```python
from build123d import *

# Parameters (mm, degrees)
SKETCH4_R               = 0.5
CUT_EXTRUDE1_DEPTH      = 60
CUT_EXTRUDE2_DEPTH      = 65.078926224
CUT_EXTRUDE2_DEPTH_BACK = 65.078926224
SKETCH5_R               = 2.5


with BuildPart() as part:
    # Sketch3 → Revolve1 (revolve)
    with BuildSketch(Plane.XY):
        with BuildLine():
            Line((-1.903971709, 4.611227449), (60.096028291, 4.611227449))
            Line((60.096028291, 4.611227449), (63.096028291, 1.611227449))
            Line((63.096028291, 1.611227449), (63.096028291, -0.388772551))
            Line((63.096028291, -0.388772551), (-6.903971709, -0.388772551))
            ThreePointArc((-6.903971709, -0.388772551), (-5.439505615, 3.146761355), (-1.903971709, 4.611227449))
        make_face()
    revolve(axis=Axis((63.096028291, -0.388772551, 0), (-1, 0, 0)))

    # Sketch4 → Cut-Extrude1 (cut)
    with BuildSketch(Plane(origin=(63.096028291, 0, 0), x_dir=(0, 0, -1), z_dir=(1, 0, 0))):
        with Locations(Location((0, -0.388772551, 0), (0, 0, 90))):
            Circle(SKETCH4_R)
    extrude(amount=-CUT_EXTRUDE1_DEPTH, mode=Mode.SUBTRACT)

    # Sketch5 → Cut-Extrude2 (cut, two sides: drawn at the far end of the back side and taken through both)
    with BuildSketch(Plane(origin=(0, 4.611227449, 0), x_dir=(1, 0, 0), z_dir=(0, 1, 0)).offset(-CUT_EXTRUDE2_DEPTH_BACK)):
        with Locations(Location((55.096028291, 0, 0), (0, 0, 180))):
            Circle(SKETCH5_R)
    extrude(amount=CUT_EXTRUDE2_DEPTH + CUT_EXTRUDE2_DEPTH_BACK, mode=Mode.SUBTRACT)


solid = part.part
```
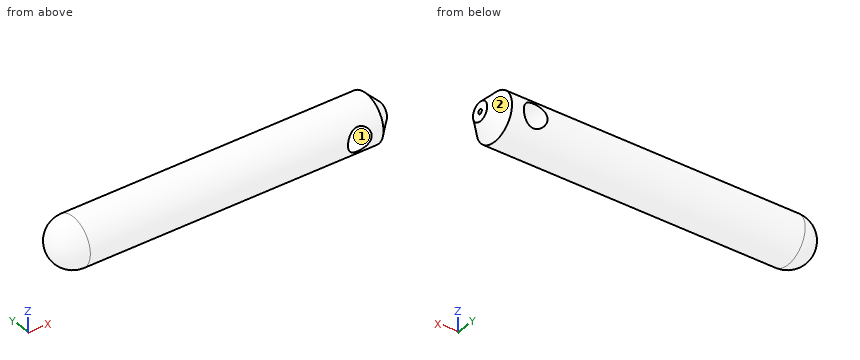
For this review, take the finished solid that the model builds, in its own axes (mm). Face numbers are marked on the shaded views. Round coordinates to 2 decimals unless told otherwise and drop trailing zeros. Write each loop counter-clockwise with the first axis right and the second up, starting at its lowest first coordinate (ties: lowest second). Pieces come first, ordered by that corner, then holes. Notation, with made-up numbers: (-3, 45) - (46, 45) arc R3 cw to (46, 50) - close; hole circle Ø1 at (18.25, 52). An arc over 180 degrees is marked (long way). Answer as a JSON object with one key per item and string values.
1. To check wall thickness, follow line 1 along Y through (x, z) = (7, 0); line 2 along X through (y, z) = (3.25, -0.25); line 3 along X through (y, z) = (2, 0.5). State the ranges of each line that lie inside material, in increasing order.
Response values:
{"line 1": "y = -5.39 to -0.89, 0.11 to 4.61", "line 2": "x = -5.32 to 52.61, 57.58 to 61.45", "line 3": "x = -6.27 to 52.65, 57.55 to 62.66"}
2. For pin 1 Ø1.5 at (x, z) = (30.5, 3.5) entering from -Y; pin 2 Ø2 at (x, z) = (45, 2.5) entering from +Y; pin 3 Ø1 at (y, z) = (-1.5, 3.5) entering from -X, all flat-tipped, find the tip position at first contact; note any pin that passes through.
Response values:
{"pin 1": "stops at y = -4.56", "pin 2": "stops at y = 4.38", "pin 3": "stops at x = -5.77"}
3. We need section A-A on x = 44. Give the boundary of the cut face in (y, z).
Response values:
{"outline": "circle Ø10 at (-0.39, 0); hole circle Ø1 at (-0.39, 0)"}
4. Draft analysis for pull direction X (two halves, no side actions). For the marked faces 1 and 2, state which applies: +X half, -X half, draft (parallel to the pull), parting line (faces both ways), or undercut.
Response values:
{"face 1": "undercut", "face 2": "+X half"}
